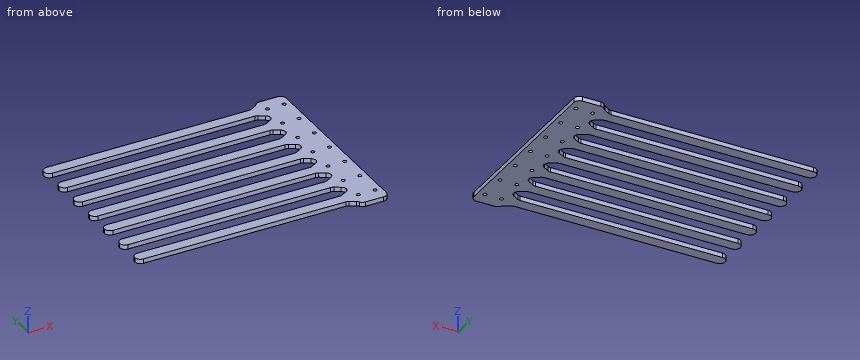
```python
from build123d import *
from OCP.BRepFilletAPI import BRepFilletAPI_MakeChamfer

# Parameters (mm, degrees)
SKETCH_1_W                  = 25
SKETCH_1_H                  = 175
EXTRUDE_1_DEPTH             = 4
SKETCH_3_R                  = 1.6
CUT_EXTRUDE_1_DEPTH         = 89.478811023
SKETCH_4_W                  = 200
SKETCH_4_H                  = 10
EXTRUDE_2_DEPTH             = 4
CHAMFER_1_SIZE              = 5
CHAMFER_1_SIZE2             = 8.660254038
FILLET_1_R                  = 5
PATTERN_LINEAR_2_DEPTH      = 4
FILLET_2_R                  = 5
PATTERN_LINEAR_3_COUNT      = 2
PATTERN_LINEAR_3_PITCH      = 15
PATTERN_LINEAR_3_COUNT_DIR2 = 7
PATTERN_LINEAR_3_PITCH_DIR2 = 25


# Read off the part's stored shape, not the designer's step: 阵列(线性)2
with BuildPart() as part:
    # 草图1 → 凸台-拉伸1 (new body)
    with BuildSketch(Plane.XY):
        Rectangle(SKETCH_1_W, SKETCH_1_H)
    extrude(amount=EXTRUDE_1_DEPTH)

    # 草图3 → 切除-拉伸1 (cut, through all)
    with BuildSketch(Plane.XY):
        with Locations((-8.5, 75)):
            Circle(SKETCH_3_R)
    cut_extrude_1 = extrude(amount=CUT_EXTRUDE_1_DEPTH, mode=Mode.SUBTRACT)

    # 草图4 → 凸台-拉伸2 (add)
    with BuildSketch(Plane.XY):
        with Locations((-110, 75)):
            Rectangle(SKETCH_4_W, SKETCH_4_H)
    extrude(amount=EXTRUDE_2_DEPTH)

    # 倒角1: one chamfer whose edges measure the first distance from different faces: ONE call of the kernel's chamfer builder (chamfer() names one face for all edges)
    chamfer_1_edges_1 = [part.edges().sort_by_distance(p)[0] for p in [
        (-12.5, 80, 2),
    ]]
    chamfer_1_side_1 = [part.faces().sort_by_distance(p)[0] for p in [
        (-12.5, 83.75, 2),
    ]]
    chamfer_1_edges_2 = [part.edges().sort_by_distance(p)[0] for p in [
        (-12.5, 70, 2),
    ]]
    chamfer_1_side_2 = [part.faces().sort_by_distance(p)[0] for p in [
        (-12.5, -8.75, 2),
    ]]
    chamfer_1 = BRepFilletAPI_MakeChamfer(part.part.solid().wrapped)
    for e in chamfer_1_edges_1:
        chamfer_1.Add(CHAMFER_1_SIZE, CHAMFER_1_SIZE2, e.wrapped, chamfer_1_side_1[0].wrapped)  # the first distance lies on this face
    for e in chamfer_1_edges_2:
        chamfer_1.Add(CHAMFER_1_SIZE, CHAMFER_1_SIZE2, e.wrapped, chamfer_1_side_2[0].wrapped)  # the first distance lies on this face
    add(Compound.cast(chamfer_1.Shape()), mode=Mode.REPLACE)

    # 圆角1
    # the kernel refuses this fillet: 5 mm, written as the material it adds along each edge
    with BuildSketch(Plane(origin=(-21.160254038, 70, 0), x_dir=(-1, 0, 0), z_dir=(0, 0, 1))) as fillet_1_piece_1:
        with BuildLine():
            CenterArc((FILLET_1_R * 0.267949192431, FILLET_1_R), FILLET_1_R, 240, 30)
            Line((-FILLET_1_R * 0.232050807569, FILLET_1_R * 0.133974596216), (0, 0))
            Line((0, 0), (FILLET_1_R * 0.267949192431, 0))
        make_face()
    extrude(amount=4)
    with BuildSketch(Plane(origin=(-12.5, 65, 0), x_dir=(0, -1, 0), z_dir=(0, 0, 1))) as fillet_1_piece_2:
        with BuildLine():
            CenterArc((FILLET_1_R * 0.57735026919, -FILLET_1_R), FILLET_1_R, 90, 60)
            Line((-FILLET_1_R * 0.288675134595, -FILLET_1_R * 0.5), (0, 0))
            Line((0, 0), (FILLET_1_R * 0.57735026919, 0))
        make_face()
    extrude(amount=4)
    with BuildSketch(Plane(origin=(-21.160254038, 80, 4), x_dir=(0.8660254037844394, 0.4999999999999988, 0), z_dir=(0, 0, -1))) as fillet_1_piece_3:
        with BuildLine():
            CenterArc((FILLET_1_R * 0.267949192431, -FILLET_1_R), FILLET_1_R, 90, 30)
            Line((-FILLET_1_R * 0.232050807569, -FILLET_1_R * 0.133974596216), (0, 0))
            Line((0, 0), (FILLET_1_R * 0.267949192431, 0))
        make_face()
    extrude(amount=4)
    with BuildSketch(Plane(origin=(-12.5, 85, 4), x_dir=(-2.0790480448337104e-12, 1.0, 0), z_dir=(0, 0, -1))) as fillet_1_piece_4:
        with BuildLine():
            CenterArc((2.895810682, -4.984308769), FILLET_1_R, 94.540406951, 55.459593049)
            Line((-1.434316336, -2.484308769), (0, 0))
            Line((0, 0), (2.5, 0))
        make_face()
    extrude(amount=4)
    # the kernel refuses this fillet: 5 mm, written as the material it takes off along each edge
    with BuildSketch(Plane(origin=(-210, 70, -12.5), x_dir=(0, 1, 0), z_dir=(0, 0, 1)), Plane(origin=(-210, 80, -12.5), x_dir=(1, 0, 0), z_dir=(0, 0, 1))) as fillet_1_2_piece_1:
        with BuildLine():
            CenterArc((FILLET_1_R, -FILLET_1_R), FILLET_1_R, 90, 90)
            Line((0, -FILLET_1_R), (0, 0))
            Line((0, 0), (FILLET_1_R, 0))
        make_face()
    extrude(amount=29, mode=Mode.SUBTRACT)

    # 阵列(线性)2 outline → 阵列(线性)2 (add)
    with BuildSketch(Plane.XY):
        with BuildLine():
            Line((-12.5, -87.5), (-12.5, -62.886751346))
            ThreePointArc((-12.5, -62.886751346), (-13.321545605, -64.919332951), (-14.933656987, -66.405072517))
            Line((-14.933656987, -66.405072517), (-20, -69.330127019))
            ThreePointArc((-20, -69.330127019), (-21.205904775, -69.829629131), (-22.5, -70))
            Line((-22.5, -70), (-205, -70))
            ThreePointArc((-205, -70), (-208.535533906, -71.464466094), (-210, -75))
            ThreePointArc((-210, -75), (-208.535533906, -78.535533906), (-205, -80))
            Line((-205, -80), (-22.5, -80))
            ThreePointArc((-22.5, -80), (-21.205904775, -80.170370869), (-20, -80.669872981))
            Line((-20, -80.669872981), (-14.984308769, -83.565683664))
            ThreePointArc((-14.984308769, -83.565683664), (-13.256610731, -85.226247178), (-12.5, -87.5))
        make_face()
        with BuildLine():
            Line((-12.5, -62.886751346), (-12.5, -37.886751346))
            ThreePointArc((-12.5, -37.886751346), (-13.321545605, -39.919332951), (-14.933656987, -41.405072517))
            Line((-14.933656987, -41.405072517), (-20, -44.330127019))
            ThreePointArc((-20, -44.330127019), (-21.205904775, -44.829629131), (-22.5, -45))
            Line((-22.5, -45), (-205, -45))
            ThreePointArc((-205, -45), (-208.535533906, -46.464466094), (-210, -50))
            ThreePointArc((-210, -50), (-208.535533906, -53.535533906), (-205, -55))
            Line((-205, -55), (-22.5, -55))
            ThreePointArc((-22.5, -55), (-21.205904775, -55.170370869), (-20, -55.669872981))
            Line((-20, -55.669872981), (-15, -58.556624327))
            ThreePointArc((-15, -58.556624327), (-13.169872981, -60.386751346), (-12.5, -62.886751346))
        make_face()
        with BuildLine():
            Line((-12.5, -37.886751346), (-12.5, -12.886751346))
            ThreePointArc((-12.5, -12.886751346), (-13.321545605, -14.919332951), (-14.933656987, -16.405072517))
            Line((-14.933656987, -16.405072517), (-20, -19.330127019))
            ThreePointArc((-20, -19.330127019), (-21.205904775, -19.829629131), (-22.5, -20))
            Line((-22.5, -20), (-205, -20))
            ThreePointArc((-205, -20), (-208.535533906, -21.464466094), (-210, -25))
            ThreePointArc((-210, -25), (-208.535533906, -28.535533906), (-205, -30))
            Line((-205, -30), (-22.5, -30))
            ThreePointArc((-22.5, -30), (-21.205904775, -30.170370869), (-20, -30.669872981))
            Line((-20, -30.669872981), (-15, -33.556624327))
            ThreePointArc((-15, -33.556624327), (-13.169872981, -35.386751346), (-12.5, -37.886751346))
        make_face()
        with BuildLine():
            Line((-12.5, -12.886751346), (-12.5, 12.113248654))
            ThreePointArc((-12.5, 12.113248654), (-13.321545605, 10.080667049), (-14.933656987, 8.594927483))
            Line((-14.933656987, 8.594927483), (-20, 5.669872981))
            ThreePointArc((-20, 5.669872981), (-21.205904775, 5.170370869), (-22.5, 5))
            Line((-22.5, 5), (-205, 5))
            ThreePointArc((-205, 5), (-208.535533906, 3.535533906), (-210, 0))
            ThreePointArc((-210, 0), (-208.535533906, -3.535533906), (-205, -5))
            Line((-205, -5), (-22.5, -5))
            ThreePointArc((-22.5, -5), (-21.205904775, -5.170370869), (-20, -5.669872981))
            Line((-20, -5.669872981), (-15, -8.556624327))
            ThreePointArc((-15, -8.556624327), (-13.169872981, -10.386751346), (-12.5, -12.886751346))
        make_face()
        with BuildLine():
            Line((-12.5, 12.113248654), (-12.5, 37.113248654))
            ThreePointArc((-12.5, 37.113248654), (-13.321545605, 35.080667049), (-14.933656987, 33.594927483))
            Line((-14.933656987, 33.594927483), (-20, 30.669872981))
            ThreePointArc((-20, 30.669872981), (-21.205904775, 30.170370869), (-22.5, 30))
            Line((-22.5, 30), (-205, 30))
            ThreePointArc((-205, 30), (-208.535533906, 28.535533906), (-210, 25))
            ThreePointArc((-210, 25), (-208.535533906, 21.464466094), (-205, 20))
            Line((-205, 20), (-22.5, 20))
            ThreePointArc((-22.5, 20), (-21.205904775, 19.829629131), (-20, 19.330127019))
            Line((-20, 19.330127019), (-15, 16.443375673))
            ThreePointArc((-15, 16.443375673), (-13.169872981, 14.613248654), (-12.5, 12.113248654))
        make_face()
        with BuildLine():
            Line((-22.5, 55), (-205, 55))
            ThreePointArc((-205, 55), (-208.535533906, 53.535533906), (-210, 50))
            ThreePointArc((-210, 50), (-208.535533906, 46.464466094), (-205, 45))
            Line((-205, 45), (-22.5, 45))
            ThreePointArc((-22.5, 45), (-21.205904775, 44.829629131), (-20, 44.330127019))
            Line((-20, 44.330127019), (-15, 41.443375673))
            ThreePointArc((-15, 41.443375673), (-13.169872981, 39.613248654), (-12.5, 37.113248654))
            Line((-12.5, 37.113248654), (-12.5, 62.113248654))
            ThreePointArc((-12.5, 62.113248654), (-13.321545605, 60.080667049), (-14.933656987, 58.594927483))
            Line((-14.933656987, 58.594927483), (-20, 55.669872981))
            ThreePointArc((-20, 55.669872981), (-21.205904775, 55.170370869), (-22.5, 55))
        make_face()
    extrude(amount=PATTERN_LINEAR_2_DEPTH)

    # 圆角2
    fillet_2_edges = [part.edges().sort_by_distance(p)[0] for p in [
        (-12.5, 87.5, 2),
        (12.5, 87.5, 2),
        (12.5, -87.5, 2),
        (-12.5, -87.5, 2),
    ]]
    fillet(fillet_2_edges, radius=FILLET_2_R)

    # 阵列(线性)3: Cut-Extrude 1 2 × 7
    with Locations(*[(i * PATTERN_LINEAR_3_PITCH, -j * PATTERN_LINEAR_3_PITCH_DIR2, 0) for i in range(PATTERN_LINEAR_3_COUNT) for j in range(PATTERN_LINEAR_3_COUNT_DIR2) if (i, j) != (0, 0)]):
        add(cut_extrude_1, mode=Mode.SUBTRACT)


solid = part.part
```
The listing builds one solid part. Answer for the finished solid, in the listing's coordinates (mm). Coordinates: 2 decimals unless noted, no trailing zeros. Order: outer loops, then holes, each group sorted by start corner. A loop starts at its lowest first (then second) coordinate and runs counter-clockwise, first axis right, second up. Notation, with made-up numbers: M 78.25,27.25 L 131.25,27.25 A26 cw 131.25,65.25 Z; hole C 60.25,45 d8. An arc over 180 degrees is marked long. Answer as a JSON object with one key per item and string values. Group by question number.
1. Section B-B on z = 0.9 is taken. State how many separate pieces and enclosed holes the cut face has, then the cut area to 3 significant figures.
2. Section A-A on x = -114 is taken. Write down the section's boundary in (y, z), then the cut area to 3 significant figures.
3. Straight lines are drawn through the part: line 1 (X direction, y = 25, z = 2.7); line 2 (X direction, y = 37, z = 1); line 3 (X direction, y = 33, z = 0.9). For each, find the intervals that lie inside material, in ascending order.
4. Flat-ended cylindrical pins translate along their axes: P1, Ø1.2, axis at x = -91, z = 2, coming from the +Y side; P2, Ø2, axis at x = -90, z = 2.5, coming from the -Y side. Find the tip coordinate at first contact, or state that the pin passes through.
Values follow:
{
 "1": {"separate pieces": "1", "enclosed holes": "14", "area": "18,300 mm2"},
 "2": {"outline": "M -80,0 L -70,0 L -70,4 L -80,4 Z; M -55,0 L -45,0 L -45,4 L -55,4 Z; M -30,0 L -20,0 L -20,4 L -30,4 Z; M -5,0 L 5,0 L 5,4 L -5,4 Z; M 20,0 L 30,0 L 30,4 L 20,4 Z; M 45,0 L 55,0 L 55,4 L 45,4 Z; M 70,0 L 80,0 L 80,4 L 70,4 Z", "area": "280 mm2"},
 "3": {"line 1": "-210 to -10.1, -6.9 to 4.9, 8.1 to 12.5", "line 2": "-12.52 to 12.5", "line 3": "-15.96 to 12.5"},
 "4": {"P1": "y = 80", "P2": "y = -80"}
}
